Autodesk Inventor part; units mm, degrees
ref_plane "YZ Plane" through (0, 0, 0) normal (1, 0, 0) x (0, 1, 0)
ref_plane "XZ Plane" through (0, 0, 0) normal (0, 1, 0) x (-1, 0, 0)
ref_plane "XY Plane" through (0, 0, 0) normal (0, 0, 1) x (1, 0, 0)
sketch "Эскиз1" plane through (0, 0, 0) normal (0, 0, 1) x (1, 0, 0)
  line L0 (0, 0) -> (20, 0)
  line L1 (20, 0) -> (20, 20)
  line L2 (20, 20) -> (0, 20)
  line L3 (0, 20) -> (0, 0)
  line L4 (1.5, 18.5) -> (18.5, 18.5)
  line L5 (18.5, 18.5) -> (18.5, 1.5)
  line L6 (18.5, 1.5) -> (1.5, 1.5)
  line L7 (1.5, 1.5) -> (1.5, 18.5)
  dimension "d0" = 1.5
  dimension "d1" = 20
  dimension "d2" = 20
extrude "Выдавливание1" add sketch "Эскиз1" along normal blind 120
sketch "Эскиз2" plane through (0, 0, 0) normal (0, -1, 0) x (1, 0, 0)
  circle A0 centre (10, 110) radius 3
  line L0 (20, 0) -> (20, 120)
  line L1 (0, 120) -> (20, 120)
  point P0 (0, 0)
  point P1 (10, 120)
  dimension "d5" = 6
  dimension "d7" = 10
extrude "Выдавливание2" cut sketch "Эскиз2" against normal through all
equation "\"d1\" = d2"
properties part number "arm"
Could you check a few things on this model? Use its own coordinates, in mm. A direction names the side the tool comes from. Round coordinates to 2 decimals unless told otherwise and drop trailing zeros. Loops run counter-clockwise (first coordinate to the right, second up) from the corner with the lowest first, then second, coordinate; pieces in that order, holes last.
Q1. I want a section at D-D (z = 110). Write out the boundary of the cut face in (x, y), and give its area (3 significant figures).
Q2. Please list where these lines run through material, in increasing order: L1, parallel to Y at x = 15.25, z = 81; L2, parallel to Z at x = 10, y = 19.25.
Q3. Thinking about a two-plate mould opening in X: for faces 3 (the cylindrical face through (12.86, 19.24, 110.9)), 4 (the flat face through (0, 10, 59)), 5 (the flat face through (1, 10, 120)), which applies, pulls with the +X half, pulls with the -X half, needs draft (parallel to the pull), parting line crosses it, or undercut?
Q4. I want a section at A-A (z = 67). Write out the boundary of the cut face in (x, y), and give its area (3 significant figures).
Q5. On a 3-axis mill with a long thin cutter (end or side, diameter ignored), from which of +Z, -Z, +X, -X, +Y, -Y can I reach the whole of each face in a straight line? I mean faces 1 (the flat face through (18.5, 10, 59)), 2 (the cylindrical face through (12.86, 0.74, 110.9)). Say none if no direction works.
Q6. I want a section at B-B (y = 3). Write out the boundary of the cut face in (x, z), and give its area (3 significant figures).
Q7. I want a section at C-C (x = 10). Write out the boundary of the cut face in (y, z).
Answer below:
1. outline: (0, 0) - (7, 0) - (7, 1.5) - (1.5, 1.5) - (1.5, 18.5) - (7, 18.5) - (7, 20) - (0, 20) - close; (13, 0) - (20, 0) - (20, 20) - (13, 20) - (13, 18.5) - (18.5, 18.5) - (18.5, 1.5) - (13, 1.5) - close
1. area: 93.0 mm2
2. L1: y = 0 to 1.5, 18.5 to 20
2. L2: z = 0 to 107, 113 to 120
3. face 3: undercut
3. face 4: pulls with the -X half
3. face 5: needs draft
4. outline: (0, 0) - (20, 0) - (20, 20) - (0, 20) - close; hole (1.5, 1.5) - (18.5, 1.5) - (18.5, 18.5) - (1.5, 18.5) - close
4. area: 111 mm2
5. face 1: +Z, -Z
5. face 2: +Y, -Y
6. outline: (0, 0) - (1.5, 0) - (1.5, 120) - (0, 120) - close; (18.5, 0) - (20, 0) - (20, 120) - (18.5, 120) - close
6. area: 360 mm2
7. outline: (0, 0) - (1.5, 0) - (1.5, 107) - (0, 107) - close; (0, 113) - (1.5, 113) - (1.5, 120) - (0, 120) - close; (18.5, 0) - (20, 0) - (20, 107) - (18.5, 107) - close; (18.5, 113) - (20, 113) - (20, 120) - (18.5, 120) - close
